```python
from build123d import *

# Parameters (mm, degrees)
SKETCH1_R           = 1.8
BOSS_EXTRUDE1_DEPTH = 10
SKETCH1_3_W         = 5
SKETCH1_3_H         = 12
BOSS_EXTRUDE2_DEPTH = 2


with BuildPart() as part:
    # Sketch1 → Boss-Extrude1 (new body)
    # profile 1 of 5: a face of its own
    with BuildSketch(Plane(origin=(0, 0, 0), x_dir=(1, 0, 0), z_dir=(0, 1, 0))):
        with BuildLine():
            Line((-52, -12), (-52, -22))
            Line((-52, -22), (-47.130495168, -24.434752416))
            Line((-47.130495168, -24.434752416), (-45.130495168, -20.434752416))
            ThreePointArc((-45.130495168, -20.434752416), (-43.223864586, -18.720952048), (-40.660607987, -18.766421636))
            Line((-40.660607987, -18.766421636), (-31.391495717, -22.605813649))
            Line((-31.391495717, -22.605813649), (-17.857864376, -17))
            Line((-17.857864376, -17), (0, -17))
            Line((0, -17), (17.857864376, -17))
            Line((17.857864376, -17), (31.391495717, -22.605813649))
            Line((31.391495717, -22.605813649), (40.660607987, -18.766421636))
            ThreePointArc((40.660607987, -18.766421636), (43.223864586, -18.720952048), (45.130495168, -20.434752416))
            Line((45.130495168, -20.434752416), (47.130495168, -24.434752416))
            Line((47.130495168, -24.434752416), (52, -22))
            Line((52, -22), (52, -12))
            Line((52, -12), (4.381103052, -3.444846378))
            ThreePointArc((4.381103052, -3.444846378), (1.5, 0), (4.381103052, 3.444846378))
            Line((4.381103052, 3.444846378), (52, 12))
            Line((52, 12), (52, 22))
            Line((52, 22), (47.130495168, 24.434752416))
            Line((47.130495168, 24.434752416), (45.130495168, 20.434752416))
            ThreePointArc((45.130495168, 20.434752416), (43.223864586, 18.720952048), (40.660607987, 18.766421636))
            Line((40.660607987, 18.766421636), (31.391495717, 22.605813649))
            Line((31.391495717, 22.605813649), (17.857864376, 17))
            Line((17.857864376, 17), (0, 17))
            Line((0, 17), (-17.857864376, 17))
            Line((-17.857864376, 17), (-31.391495717, 22.605813649))
            Line((-31.391495717, 22.605813649), (-40.660607987, 18.766421636))
            ThreePointArc((-40.660607987, 18.766421636), (-43.223864586, 18.720952048), (-45.130495168, 20.434752416))
            Line((-45.130495168, 20.434752416), (-47.130495168, 24.434752416))
            Line((-47.130495168, 24.434752416), (-52, 22))
            Line((-52, 22), (-52, 12))
            Line((-52, 12), (-4.381103052, 3.444846378))
            ThreePointArc((-4.381103052, 3.444846378), (-1.5, 0), (-4.381103052, -3.444846378))
            Line((-4.381103052, -3.444846378), (-52, -12))
        make_face()
    # profile 2 of 5: a face of its own
    with BuildSketch(Plane(origin=(0, 0, 0), x_dir=(1, 0, 0), z_dir=(0, 1, 0))):
        with BuildLine():
            Line((-42, 27), (-47.130495168, 24.434752416))
            Line((-47.130495168, 24.434752416), (-45.130495168, 20.434752416))
            ThreePointArc((-45.130495168, 20.434752416), (-43.223864586, 18.720952048), (-40.660607987, 18.766421636))
            Line((-40.660607987, 18.766421636), (-31.391495717, 22.605813649))
            Line((-31.391495717, 22.605813649), (-42, 27))
        make_face()
        with Locations(Location((-42, 22, 0), (0, 0, 270))):
            Circle(SKETCH1_R, mode=Mode.SUBTRACT)
    # profile 3 of 5: a face of its own
    with BuildSketch(Plane(origin=(0, 0, 0), x_dir=(1, 0, 0), z_dir=(0, 1, 0))):
        with BuildLine():
            Line((-47.130495168, -24.434752416), (-42, -27))
            Line((-42, -27), (-31.391495717, -22.605813649))
            Line((-31.391495717, -22.605813649), (-40.660607987, -18.766421636))
            ThreePointArc((-40.660607987, -18.766421636), (-43.223864586, -18.720952048), (-45.130495168, -20.434752416))
            Line((-45.130495168, -20.434752416), (-47.130495168, -24.434752416))
        make_face()
        with Locations(Location((-42, -22, 0), (0, 0, 270))):
            Circle(SKETCH1_R, mode=Mode.SUBTRACT)
    # profile 4 of 5: a face of its own
    with BuildSketch(Plane(origin=(0, 0, 0), x_dir=(1, 0, 0), z_dir=(0, 1, 0))):
        with BuildLine():
            Line((47.130495168, 24.434752416), (42, 27))
            Line((42, 27), (31.391495717, 22.605813649))
            Line((31.391495717, 22.605813649), (40.660607987, 18.766421636))
            ThreePointArc((40.660607987, 18.766421636), (43.223864586, 18.720952048), (45.130495168, 20.434752416))
            Line((45.130495168, 20.434752416), (47.130495168, 24.434752416))
        make_face()
        with Locations(Location((42, 22, 0), (0, 0, 270))):
            Circle(SKETCH1_R, mode=Mode.SUBTRACT)
    # profile 5 of 5: a face of its own
    with BuildSketch(Plane(origin=(0, 0, 0), x_dir=(1, 0, 0), z_dir=(0, 1, 0))):
        with BuildLine():
            Line((31.391495717, -22.605813649), (42, -27))
            Line((42, -27), (47.130495168, -24.434752416))
            Line((47.130495168, -24.434752416), (45.130495168, -20.434752416))
            ThreePointArc((45.130495168, -20.434752416), (43.223864586, -18.720952048), (40.660607987, -18.766421636))
            Line((40.660607987, -18.766421636), (31.391495717, -22.605813649))
        make_face()
        with Locations(Location((42, -22, 0), (0, 0, 270))):
            Circle(SKETCH1_R, mode=Mode.SUBTRACT)
    extrude(amount=BOSS_EXTRUDE1_DEPTH)

    # Sketch1_3 → Boss-Extrude2 (add)
    # profile 1 of 2: a face of its own
    with BuildSketch(Plane(origin=(0, 0, 0), x_dir=(1, 0, 0), z_dir=(0, 1, 0))):
        with BuildLine():
            Line((-52, 12), (-52, -12))
            Line((-52, -12), (-4.381103052, -3.444846378))
            ThreePointArc((-4.381103052, -3.444846378), (-1.5, 0), (-4.381103052, 3.444846378))
            Line((-4.381103052, 3.444846378), (-52, 12))
        make_face()
        with Locations((-39.5, 0)):
            Rectangle(SKETCH1_3_W, SKETCH1_3_H, mode=Mode.SUBTRACT)
    # profile 2 of 2: a face of its own
    with BuildSketch(Plane(origin=(0, 0, 0), x_dir=(1, 0, 0), z_dir=(0, 1, 0))):
        with BuildLine():
            Line((4.381103052, -3.444846378), (52, -12))
            Line((52, -12), (52, 12))
            Line((52, 12), (4.381103052, 3.444846378))
            ThreePointArc((4.381103052, 3.444846378), (1.5, 0), (4.381103052, -3.444846378))
        make_face()
        with Locations((39.5, 0)):
            Rectangle(SKETCH1_3_W, SKETCH1_3_H, mode=Mode.SUBTRACT)
    extrude(amount=BOSS_EXTRUDE2_DEPTH)


solid = part.part
```
Work out the finished part from the listing and answer in its coordinate system (mm). A direction names the side the tool comes from. Coordinates: 2 decimals unless noted, no trailing zeros. Write each loop counter-clockwise with the first axis right and the second up, starting at its lowest first coordinate (ties: lowest second). Pieces come first, ordered by that corner, then holes.
Q1. Each of these flat-tipped pins is pushed along its axis until it touches: pin 1 Ø2 at (x, z) = (-42, 22) entering from -Y; pin 2 Ø1 at (x, y) = (-8.5, 4.5) entering from -Z; pin 3 Ø4 at (x, z) = (-42, -22) entering from +Y; pin 4 Ø1.6 at (x, y) = (-40.5, 1) entering from -Z. Where does it stop, or does it pass through?
Q2. A cutting plane is placed at C-C, the plane z = 19. Give the vertices of the cut face in (x, y).
Q3. Which of the six approach directions +Z, -Z, +X, -X, +Y, -Y give full straight-line access (tool end or side, diameter ignored) to faces 1 (the face through (47.07, 4.93, -24.465)), 2 (the face through (-40, 1, -6)), 3 (the face through (0, 5, 17)), 4 (the face through (-33, 2, 0)), 5 (the face through (27.857, 5.944, -7.663))?
Q4. A cutting plane is placed at D-D, the plane x = -20. Give the vertices of the cut face in (y, z).
Q5. A cutting plane is placed at A-A, the plane y = 5.25. Give the vertices of the cut face in (x, z).
Q6. Find the intervals of material crossed by line 1 (X direction, y = 1.5, z = -4); line 2 (Z direction, x = -9.5, y = 7); line 3 (X direction, y = 5.5, z = 22), in increasing order.
Q7. A cutting plane is placed at B-B, the plane z = -0.5. Give the vertices of the cut face in (x, y).
Q8. Determine the mould class of faces 6 (the face through (52, 1.6, 0.3)), 7 (the face through (-46.93, 4.93, -24.535)), 8 (the face through (32, 2, 0)) for opening direction Z: released by +Z, released by -Z, zero draft, split by the parting line, or undercut.
Findings below:
1. pin 1: passes through
1. pin 2: stops at z = -17
1. pin 3: stops at y = 10
1. pin 4: stops at z = -26.71
2. outline: (-52, 0) - (-22.69, 0) - (-22.69, 10) - (-52, 10) - close; (22.69, 0) - (52, 0) - (52, 10) - (22.69, 10) - close
3. face 1: -Z, +X, +Y, -Y
3. face 2: +Y, -Y
3. face 3: +Z, +Y, -Y
3. face 4: -X, +Y
3. face 5: +X, +Y
4. outline: (0, -17.89) - (10, -17.89) - (10, -6.25) - (2, -6.25) - (2, 6.25) - (10, 6.25) - (10, 17.89) - (0, 17.89) - close
5. outline: (-52, -22) - (-42, -27) - (-17.86, -17) - (17.86, -17) - (42, -27) - (52, -22) - (52, -12) - (4.38, -3.44) arc R3.5 cw to (4.38, 3.44) - (52, 12) - (52, 22) - (42, 27) - (17.86, 17) - (-17.86, 17) - (-42, 27) - (-52, 22) - (-52, 12) - (-4.38, 3.44) arc R3.5 cw to (-4.38, -3.44) - (-52, -12) - close; hole circle Ø3.6 at (-42, -22); hole circle Ø3.6 at (-42, 22); hole circle Ø3.6 at (42, -22); hole circle Ø3.6 at (42, 22)
6. line 1: x = -52 to -42, -37 to 37, 42 to 52
6. line 2: z = -17 to -4.36, 4.36 to 17
6. line 3: x = -52 to -43.8, -40.2 to -29.93, 29.93 to 40.2, 43.8 to 52
7. outline: (-52, 0) - (-42, 0) - (-42, 2) - (-52, 2) - close; (-37, 0) - (37, 0) - (37, 2) - (1.54, 2) - (1.54, 10) - (-1.54, 10) - (-1.54, 2) - (-37, 2) - close; (42, 0) - (52, 0) - (52, 2) - (42, 2) - close
8. face 6: zero draft
8. face 7: released by -Z
8. face 8: undercut
